Source: CAD feature listing. Evaluate the final solid. Frame: model axes, mm. A direction names the side the tool comes from. Round coordinates to 2 decimals unless told otherwise and drop trailing zeros. Loops run counter-clockwise (first coordinate to the right, second up) from the corner with the lowest first, then second, coordinate; pieces in that order, holes last.
Item 1: Ray query, L1, parallel to X at y = -11.2, z = 0; L2, parallel to Y at x = 0, z = 4.75; L3, parallel to Y at x = 0, z = -1. Return the intervals inside material, ascending.
Item 2: Section query C-C on z = 3. Return loops of the section in (x, y).
Item 3: Access query for faces 1 (the cylindrical face through (6.586, 10.329, 4.76)), 2 (the cylindrical face through (22.43, -11.04, 5.4)), 3 (the flat face through (16.6, -8.5, -1.2)), 4 (the flat face through (-13.32, -10.8, 4.03)), 5 (the flat face through (-6, -13, -2)). Directions: +Z, -Z, +X, -X, +Y, -Y. A direction counts if a zero-diameter tool reaches every point of the face in a straight line with its end or side. Return the directions, or none.
Item 4: Pull-direction query (X, two-part tool) for faces 6 (the cylindrical face through (6.586, -10.329, -4.74)), 7 (the cylindrical face through (-22.4, -10.96, -5.43)), 8 (the flat face through (23, -11, 0)); classes: released by +X, released by -X, zero draft, split by the parting line, or undercut.
Item 5: Section query B-B on z = 0. Return loops of the section in (x, y).
Item 6: First-contact query: P1, Ø12, axis at x = -2.5, y = -4, coming from the -Z side; P2, Ø1, axis at x = -7.5, z = -4.5, coming from the +Y side; P3, Ø2.5, axis at x = -18.5, z = -1, coming from the +Y side; P4, Ø6, axis at y = 3, z = 1.5, coming from the -X side. Flat tips, straight axial feed; report the tip coordinate or a pass-through.
```python
from build123d import *

# Parameters (mm, degrees)
CROQUIS1_R              = 11
SALIENTE_EXTRUIR1_DEPTH = 6
CROQUIS2_R              = 2
CORTAR_EXTRUIR1_DEPTH   = 33.388269481
CORTAR_EXTRUIR2_DEPTH   = 30.244657632
SALIENTE_EXTRUIR2_DEPTH = 2
CROQUIS6_R              = 12.25
CORTAR_EXTRUIR3_DEPTH   = 2
CORTAR_EXTRUIR4_START   = -2
CROQUIS7_R              = 12.25
CORTAR_EXTRUIR4_DEPTH   = 2
REDONDEO1_R             = 2
REDONDEO2_R             = 2
REDONDEO3_R             = 2
REDONDEO4_R             = 0.5


with BuildPart() as part:
    # Croquis1 → Saliente-Extruir1 (new, symmetric)
    with BuildSketch(Plane.XY):
        with BuildLine():
            Line((23, -13.5), (-23, -13.5))
            Line((-23, -13.5), (-23, -8.5))
            Line((-23, -8.5), (-14.237940292, -8.5))
            Line((-14.237940292, -8.5), (-13.5, 0))
            ThreePointArc((-13.5, 0), (0, 13.5), (13.5, 0))
            Line((13.5, 0), (14.237940292, -8.5))
            Line((14.237940292, -8.5), (23, -8.5))
            Line((23, -8.5), (23, -13.5))
        make_face()
        Circle(CROQUIS1_R, mode=Mode.SUBTRACT)
    extrude(amount=SALIENTE_EXTRUIR1_DEPTH, both=True)

    # Croquis2 → Cortar-Extruir1 (cut, through all)
    with BuildSketch(Plane(origin=(0, -8.5, 0), x_dir=(1, 0, 0), z_dir=(0, 1, 0))):
        with Locations(Location((-18.618970146, 0, 0), (0, 0, 270))):
            Circle(CROQUIS2_R)
        with Locations(Location((18.618970146, 0, 0), (0, 0, 90))):
            Circle(CROQUIS2_R)
    extrude(amount=-CORTAR_EXTRUIR1_DEPTH, mode=Mode.SUBTRACT)

    # Croquis3 → Cortar-Extruir2 (cut, through all)
    with BuildSketch(Plane.XY.offset(6)):
        with BuildLine():
            Line((-13.553865986, -13.5), (13.553865986, -13.5))
            Line((13.553865986, -13.5), (13.090777783, -8.165896733))
            ThreePointArc((13.090777783, -8.165896733), (11.758860153, -7.768821091), (10.539573747, -8.435915012))
            ThreePointArc((10.539573747, -8.435915012), (0, -13.499899143), (-10.539573747, -8.435915012))
            ThreePointArc((-10.539573747, -8.435915012), (-11.758860153, -7.768821091), (-13.090777783, -8.165896733))
            Line((-13.090777783, -8.165896733), (-13.553865986, -13.5))
        make_face()
    extrude(amount=-CORTAR_EXTRUIR2_DEPTH, mode=Mode.SUBTRACT)

    # Croquis5 → Saliente-Extruir2 (add, symmetric)
    with BuildSketch(Plane.XY):
        Polygon((-13.553865986, -13.5), (13.553865986, -13.5), (13.090777783, -8.165896733), (11.052644105, -6.744861607), (3.381214515, -12.283091016), (-4.357609146, -12.066622794), (-11.573003147, -6.744861607), (-13.322321885, -7.45537917), align=None)
    extrude(amount=SALIENTE_EXTRUIR2_DEPTH, both=True)

    # Croquis6 → Cortar-Extruir3 (cut)
    with BuildSketch(Plane.XY.offset(6)):
        Circle(CROQUIS6_R)
    extrude(amount=-CORTAR_EXTRUIR3_DEPTH, mode=Mode.SUBTRACT)

    # Croquis7 → Cortar-Extruir4 (cut)
    with BuildSketch(Plane(origin=(0, 0, -6), x_dir=(-1, 0, 0), z_dir=(0, 0, -1)).offset(CORTAR_EXTRUIR4_START)):
        with Locations(Location((0, 0, 0), (0, 0, 180))):
            Circle(CROQUIS7_R)
    extrude(amount=CORTAR_EXTRUIR4_DEPTH, mode=Mode.SUBTRACT)

    # Redondeo1
    redondeo1_edges = [part.edges().sort_by_distance(p)[0] for p in [
        (23, -11, -6),
    ]]
    fillet(redondeo1_edges, radius=REDONDEO1_R)

    # Redondeo2
    redondeo2_edges = [part.edges().sort_by_distance(p)[0] for p in [
        (23, -11, 6),
    ]]
    fillet(redondeo2_edges, radius=REDONDEO2_R)

    # Redondeo3
    redondeo3_edges = [part.edges().sort_by_distance(p)[0] for p in [
        (-23, -11, -6),
        (-23, -11, 6),
    ]]
    fillet(redondeo3_edges, radius=REDONDEO3_R)

    # Redondeo4
    redondeo4_edges = [part.edges().sort_by_distance(p)[0] for p in [
        (-12.25, 0, -6),
        (-12.25, 0, 6),
    ]]
    fillet(redondeo4_edges, radius=REDONDEO4_R)


solid = part.part
```
Data:
1. L1: x = -23 to -20.62, -16.62 to 16.62, 20.62 to 23
1. L2: y = -13.5 to -12.25, 12.25 to 13.5
1. L3: y = -13.5 to -11, 11 to 13.5
2. outline: (-23, -13.5) - (-13.55, -13.5) - (-13.09, -8.17) arc R1.81 cw to (-10.54, -8.44) arc R13.5 ccw to (10.54, -8.44) arc R1.81 cw to (13.09, -8.17) - (13.55, -13.5) - (23, -13.5) - (23, -8.5) - (14.24, -8.5) - (13.5, 0) arc R13.5 ccw to (-13.5, 0) - (-14.24, -8.5) - (-23, -8.5) - close; hole circle Ø22 at (0, 0)
3. face 1: +Z
3. face 2: +Z, +X, +Y, -Y
3. face 3: +Z, -Z, +X, +Y
3. face 4: +Z, -Y
3. face 5: -Z, -Y
4. face 6: undercut
4. face 7: released by -X
4. face 8: released by +X
5. outline: (-23, -13.5) - (-20.62, -13.5) - (-20.62, -8.5) - (-23, -8.5) - close; (-16.62, -13.5) - (16.62, -13.5) - (16.62, -8.5) - (14.24, -8.5) - (13.5, 0) arc R13.5 ccw to (-13.5, 0) - (-14.24, -8.5) - (-16.62, -8.5) - close; (20.62, -13.5) - (23, -13.5) - (23, -8.5) - (20.62, -8.5) - close; hole circle Ø22 at (0, 0); hole (12.87, -8.01) - (13.09, -8.17) arc R1.81 ccw to start
6. P1: passes through
6. P2: stops at y = 11.54
6. P3: stops at y = -8.5
6. P4: stops at x = -13.5
